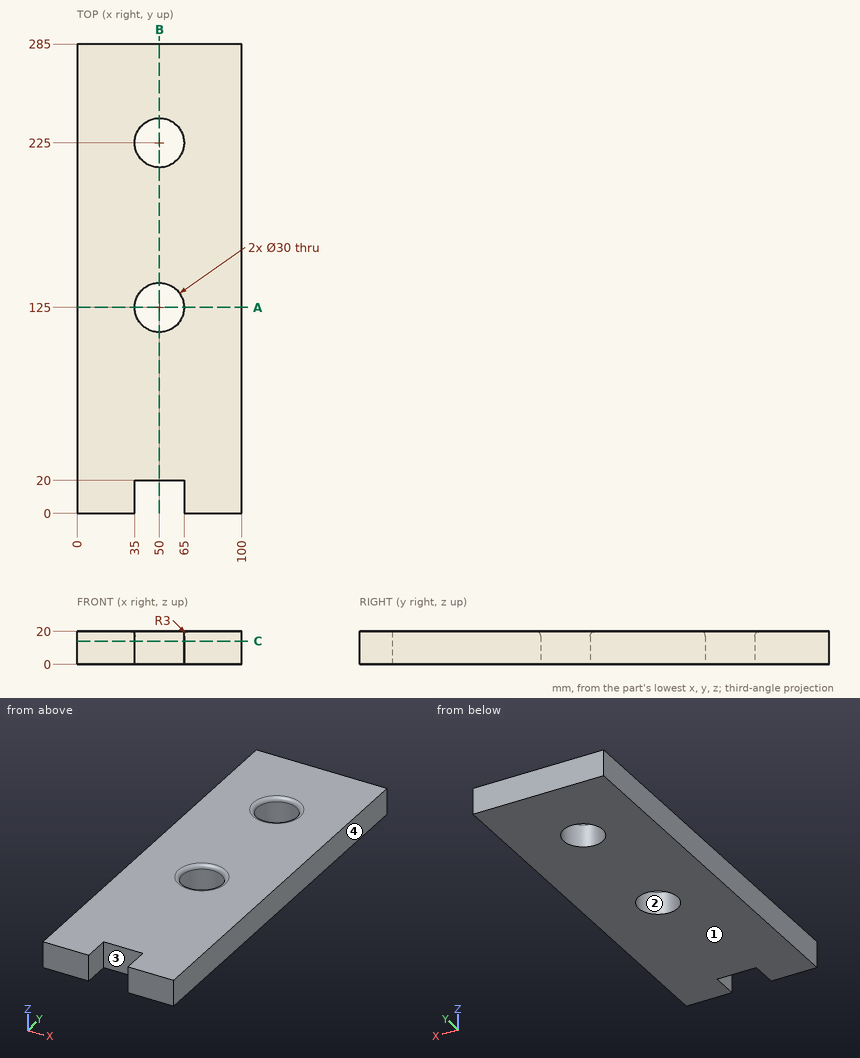
Design review of the part shown in the three views and the two pictorial views. Dimensions are in mm from the part's minimum x, y and z. Coordinates: 2 decimals unless noted, no trailing zeros. Loops run counter-clockwise (first coordinate to the right, second up) from the corner with the lowest first, then second, coordinate; pieces in that order, holes last. Notation, with made-up numbers: M 26,45 L 74,45 A13 cw 74,60 Z; hole C -10,64.5 d6. An arc over 180 degrees is marked long. One line per question, with ' | ' between items.
(1) Wall thickness on probe 1 along Y at (x, z) = (50, 10.75); probe 2 along Y at (x, z) = (41.5, 11.25); probe 3 along X at (y, z) = (228, 3.5): over which ranges is each line inside the solid? List them lowest first.
Filled in:
probe 1: y = 20 to 110, 140 to 210, 240 to 285 | probe 2: y = 20 to 112.64, 137.36 to 212.64, 237.36 to 285 | probe 3: x = 0 to 35.3, 64.7 to 100
(2) Draft analysis for pull direction X (two halves, no side actions). For the marked faces 1, 2, 3 and 4, state which applies: released by +X, released by -X, zero draft, split by the parting line, or undercut.
Filled in:
face 1: zero draft | face 2: undercut | face 3: undercut | face 4: released by +X
(3) For pin 1 Ø18 at (x, y) = (50, 225) entering from -Z; pin 2 Ø6 at (x, z) = (49.5, 5.5) entering from -Y, all flat-tipped, find the tip position at first contact; note any pin that passes through.
Filled in:
pin 1: passes through | pin 2: stops at y = 20
(4) We need section A-A (y = 125). Give the boundary of the cut face in (x, z).
Filled in:
outline: M 0,0 L 35,0 L 35,17 A3 ccw 32,20 L 0,20 Z; M 65,0 L 100,0 L 100,20 L 68,20 A3 ccw 65,17 Z
(5) We need section C-C (z = 14). Give the boundary of the cut face in (x, y), and give its area (3 significant figures).
Filled in:
outline: M 0,0 L 35,0 L 35,20 L 65,20 L 65,0 L 100,0 L 100,285 L 0,285 Z; hole C 50,125 d30; hole C 50,225 d30 | area: 26,500 mm^2
(6) We need section B-B (x = 50). Give the boundary of the cut face in (y, z), and give its area (3 significant figures).
Filled in:
outline: M 20,0 L 110,0 L 110,17 A3 ccw 107,20 L 20,20 Z; M 140,0 L 210,0 L 210,17 A3 ccw 207,20 L 143,20 A3 ccw 140,17 Z; M 240,0 L 285,0 L 285,20 L 243,20 A3 ccw 240,17 Z | area: 4,090 mm^2
